The listing builds one solid part. Answer for the finished solid, in the listing's coordinates (mm). A direction names the side the tool comes from. Round coordinates to 2 decimals unless told otherwise and drop trailing zeros. Loops run counter-clockwise (first coordinate to the right, second up) from the corner with the lowest first, then second, coordinate; pieces in that order, holes last. Notation, with made-up numbers: (-35, -5.5) -> (4, -5.5) arc R28 cw to (4, 16.5) -> close; hole circle Ø6 at (-14, 16). An arc over 180 degrees is marked (long way). Answer in a Markdown table with one row per item. Add a question column.
Autodesk Inventor part; units mm, degrees
ref_plane "Work Plane12" through (0, 0, 0) normal (0, 1, 0) x (1, 0, 0)
ref_plane "Work Plane7" through (0, 5, 0) normal (0, 1, 0) x (1, 0, 0)
ref_plane "Work Plane6" through (0, 5, 0) normal (0, 1, 0) x (1, 0, 0)
ref_plane "Work Plane12" through (0, 0, 0) normal (0, 1, 0) x (1, 0, 0)
sketch "Sketch2" plane through (0, 0, 0) normal (0, 1, 0) x (1, 0, 0)
  line L0 (-10, -65) -> (-10, -85)
  line L1 (-10, -85) -> (20, -85)
  line L2 (-10, -50) -> (-10, -15)
  line L3 (17.5697, -20.0796) -> (74.4447, -85.0796) construction
  line L4 (80.25, -80) -> (80.25, -36.3042) construction
  line L5 (-10, -65) -> (-10, -50)
  arc A0 (80.25, -80) -> (23.375, -15) centre (15.252, -79.4904) ccw
  line L6 (20, -85) -> (20, -15)
  line L7 (20, -85) -> (90, -85) construction
  line L8 (20, -15) -> (-10, -15)
  point P0 (0, -80)
  point P1 (0, 0)
  dimension "d13" = 30
  dimension "d14" = 20
  dimension "d15" = 35
  dimension "d98" = 70
  dimension "d99" = 90
extrude "Extrusion2" add sketch "Sketch2" along normal blind 5
ref_plane "Work Plane7" through (0, 5, 0) normal (0, 1, 0) x (1, 0, 0)
ref_plane "Work Plane6" through (0, 5, 0) normal (0, 1, 0) x (1, 0, 0)
sketch "Sketch7" plane through (0, 5, 0) normal (0, 1, 0) x (1, 0, 0)
  line L0 (-2.5, -32.5) -> (7.5, -32.5)
  line L1 (2.5, -32.5) -> (15, -75.625) construction
  line L2 (15, -85) -> (15, -65)
  line L3 (-2.5, -45) -> (7.5, -45)
  line L4 (2.5, -45) -> (2.5, -70) construction
  line L5 (2.5, -57.5) -> (-13.1217, -57.5) construction
  point P0 (0, 0)
  point P1 (20, -85)
  dimension "d54" = 25
ref_plane "Work Plane8" through (-2.5, 5, 45) normal (0, 0, 1) x (1, 0, 0)
sketch "Sketch8" plane through (-2.5, 5, 45) normal (0, 0, 1) x (1, 0, 0)
  line L0 (-7.5, 0) -> (22.5, 0)
  arc A0 (22.5, 18) -> (-7.5, 18) centre (7.5, 18) ccw
  line L1 (-7.5, 18) -> (-7.5, 0)
  line L2 (22.5, 18) -> (22.5, 0)
  point P0 (2.5, -5)
  dimension "d100" = 30
extrude "Extrusion7" add sketch "Sketch8" against normal blind 15
ref_plane "Work Plane9" through (-2.5, 5, 45) normal (0, 0, 1) x (1, 0, 0)
sketch "Sketch9" plane through (-2.5, 5, 45) normal (0, 0, 1) x (1, 0, 0)
  arc A0 (-2, 18) -> (17, 18) centre (7.5, 18) ccw
  line L0 (-2, 18) -> (-2, 26.124)
  line L1 (17, 18) -> (17, 26.124)
  line L2 (22.5, 0) -> (-7.5, 0) construction
  line L3 (7.5, 0) -> (7.5, 18) construction
  arc A1 (22.5, 18) -> (-7.5, 18) centre (7.5, 18) ccw construction
  line L4 (17, 26.124) -> (20.1095, 26.124)
  line L5 (-2, 26.124) -> (-5.1095, 26.124)
  arc A2 (20.1095, 26.124) -> (-5.1095, 26.124) centre (7.5, 18) ccw
  point P0 (2.5, -5)
  dimension "d47" = 19
extrude "Extrusion8" cut sketch "Sketch9" against normal blind 10
ref_plane "Work Plane10" through (2.5, 23, 30) normal (0, 0, -1) x (-1, 0, 0)
sketch "Sketch10" plane through (2.5, 23, 30) normal (0, 0, -1) x (-1, 0, 0)
  line L0 (-5, 0) -> (5, 0)
  arc A0 (-12, 0) -> (7, 0) centre (-2.5, 0) ccw
  circle A1 centre (-2.5, 0) radius 4
  point P0 (2.5, -23)
  dimension "d103" = 8
extrude "Extrusion9" cut sketch "Sketch10" against normal blind 5
ref_plane "Work Plane2" through (2.5, 5, 57.5) normal (0, 0, 1) x (1, 0, 0)
mirror "Mirror2" about plane through (2.5, 5, 57.5) normal (0, 0, 1) of "Extrusion7", "Extrusion8", "Extrusion9"
ref_plane "Work Plane11" through (2.5, 23, 85) normal (0, 0, 1) x (1, 0, 0)
sketch "Sketch11" plane through (2.5, 23, 85) normal (0, 0, 1) x (1, 0, 0)
  line L0 (-12.5, 20) -> (17.5, 20)
  line L1 (17.5, 20) -> (17.5, 10)
  line L2 (17.5, 10) -> (-12.5, 10)
  line L3 (-12.5, 10) -> (-12.5, 20)
  arc A0 (17.5, 0) -> (-12.5, 0) centre (2.5, 0) ccw
  line L4 (-12.5, 20) -> (17.5, 10) construction
  line L5 (17.5, 20) -> (-12.5, 10) construction
  point P0 (-2.5, -23)
  point P1 (2.5, 15)
  dimension "d101" = 30
  dimension "d102" = 10
extrude "Extrusion10" cut sketch "Sketch11" against normal blind 80
ref_plane "Work Plane14" through (0, 0, 0) normal (0, -1, 0) x (1, 0, 0)
sketch "Sketch17" plane through (0, 0, 0) normal (0, -1, 0) x (1, 0, 0)
  line L0 (15, 15) -> (-10, 15)
  line L1 (-10, 15) -> (15, 15)
  line L2 (-10, 15) -> (-10, 30)
  line L3 (-10, 15) -> (-10, 85)
  line L4 (-10, 85) -> (80, 85)
  arc A0 (15, 15) -> (80, 85) centre (15, 80.1786) ccw
  point P0 (0, 0)
  dimension "d94" = 90
extrude "Extrusion16" add sketch "Sketch17" along normal blind 5
sketch "Sketch18" plane through (0, 0, 0) normal (0, 1, 0) x (1, 0, 0)
  line L0 (20, -70) -> (20, -45) construction
  line L1 (20, -57.5) -> (60, -57.5) construction
  line L2 (20, -57.5) -> (30, -57.5) construction
  line L3 (30, -57.5) -> (30, -37.5) construction
  line L4 (30, -57.5) -> (30, -77.5) construction
  circle A0 centre (30, -67.5) radius 5
  circle A1 centre (30, -47.5) radius 5
  circle A2 centre (60, -57.5) radius 5
  point P0 (0, 0)
  dimension "d104" = 40
  dimension "d105" = 10
  dimension "d106" = 20
  dimension "d107" = 20
  dimension "d108" = 10
  dimension "d109" = 10
  dimension "d110" = 10
extrude "Extrusion17" cut sketch "Sketch18" against normal blind 5
properties part number "beta_plate"
Item 1: Section C-C, the plane z = 47.5 is taken. Write down the section's boundary in (x, y), and give its area (3 significant figures).
Item 2: Flat-ended cylindrical pins translate along their axes: P1, Ø6, axis at x = 60, z = 57.5, coming from the +Y side; P2, Ø13, axis at x = 5, y = 23, coming from the -Z side; P3, Ø3.5, axis at x = -5.5, z = 39, coming from the +Y side; P4, Ø18.5, axis at y = 12, z = 34, coming from the +X side. Find the tip coordinate at first contact, or state that the pin passes through.
Item 3: Consider L1, parallel to Z at x = 30, y = -3; L2, parallel to Y at x = 5, z = 81.75; L3, parallel to Z at x = 17.5, y = 28. Determine where each line is inside the solid, lowest interval first. Write a range as from..to.
Item 4: Section A-A, the plane x = 5 is taken. Write down the section's boundary in (y, z).
Item 5: Section B-B, the plane y = 6.5 is taken. Write down the section's boundary in (x, z), and give its area (3 significant figures).
Item 6: For faces 1 (the flat face through (5, 12, 45)), 2 (the flat face through (14.5, 27, 40)), 3 (the flat face through (24, -5, 50)), 4 (the flat face through (43, 0, 58)), 5 (the cylindrical face through (-9.42, 27.13, 77.4)), determine the directions among +Z, -Z, +X, -X, +Y, -Y from which every point of the face is accessible in a straight line to the end or side of a thin tool.
Item 7: Section D-D, the plane x = 60 is taken. Write down the section's boundary in (y, z), and give its area (3 significant figures).
Here are the results:
| question | item | result |
|---|---|---|
| 1 | outline | (-10, -5) -> (25, -5) -> (25, 0) -> (20, 0) -> (20, 5) -> (-10, 5) -> close; (35, -5) -> (71.39, -5) -> (71.39, 0) -> (35, 0) -> close |
| 1 | area | 507 mm² |
| 2 | P1 | passes through |
| 2 | P2 | stops at z = 30 |
| 2 | P3 | stops at y = 31.12 |
| 2 | P4 | stops at x = 20 |
| 3 | L1 | z = 16.75..42.5, 52.5..62.5, 72.5..85 |
| 3 | L2 | y = -5..19, 27..33 |
| 3 | L3 | z = 30..45, 70..85 |
| 4 | outline | (-5, 15) -> (5, 15) -> (5, 30) -> (19, 30) -> (19, 35) -> (13.5, 35) -> (13.5, 45) -> (5, 45) -> (5, 70) -> (13.5, 70) -> (13.5, 80) -> (19, 80) -> (19, 85) -> (-5, 85) -> close; (27, 30) -> (33, 30) -> (33, 35) -> (27, 35) -> close; (27, 80) -> (33, 80) -> (33, 85) -> (27, 85) -> close |
| 5 | outline | (-10, 30) -> (20, 30) -> (20, 45) -> (-10, 45) -> close; (-10, 70) -> (20, 70) -> (20, 85) -> (-10, 85) -> close |
| 5 | area | 900 mm² |
| 6 | face 1 | +X, -X, +Y |
| 6 | face 2 | +Y |
| 6 | face 3 | +Z, -Z, +X, -X, -Y |
| 6 | face 4 | +Z, -Z, +X, +Y |
| 6 | face 5 | +Z, -Z, -X, +Y |
| 7 | outline | (-5, 33.03) -> (0, 33.03) -> (0, 52.5) -> (-5, 52.5) -> close; (-5, 62.5) -> (0, 62.5) -> (0, 85) -> (-5, 85) -> close |
| 7 | area | 210 mm² |
